The model under review builds one solid part; all positions refer to its coordinate system, in mm. A direction names the side the tool comes from. Give positions to 0.01 mm unless a question says otherwise; leave off trailing zeros. Loops run counter-clockwise (first coordinate to the right, second up) from the corner with the lowest first, then second, coordinate; pieces in that order, holes last. Notation, with made-up numbers: M 21,70 L 46,70 A18 cw 46,87 Z; hole C 14.25,-29.75 d9. An arc over 180 degrees is marked long. Return JSON: item names as keys, results as strings.
```python
from build123d import *

# Parameters (mm, degrees)
SKETCH1_W                       = 112
SKETCH1_H                       = 35.5
BOSS_EXTRUDE1_DEPTH             = 1.2
SKETCH2_W                       = 6
SKETCH2_H                       = 6
BOSS_EXTRUDE2_DEPTH             = 2
SKETCH3_R                       = 1.1
CUT_EXTRUDE1_DEPTH              = 59.83283522
SKETCH5_W                       = 20
SKETCH5_H                       = 14
CUT_EXTRUDE3_DEPTH              = 59.83283522
CHAMFER1_SIZE                   = 0.4
CUT_EXTRUDE6_DEPTH              = 59.779779687
CUT_EXTRUDE6_DEPTH_BACK         = 59.779779687
SKETCH8_W                       = 0.4
SKETCH8_H                       = 35.5
SKIZZE1_W                       = 5.6
SKIZZE1_H                       = 23.5
AUFSATZ_LINEAR_AUSTRAGEN1_DEPTH = 2
SKETCH9_W                       = 5.6
SKETCH9_H                       = 35.5
CUT_EXTRUDE7_DEPTH              = 2
CHAMFER2_SIZE                   = 1.3


with BuildPart() as part:
    # Sketch1 → Boss-Extrude1 (new body)
    with BuildSketch(Plane.XY):
        Rectangle(SKETCH1_W, SKETCH1_H)
    extrude(amount=BOSS_EXTRUDE1_DEPTH)

    # Sketch2 → Boss-Extrude2 (add)
    with BuildSketch(Plane.XY.offset(1.2)):
        with Locations((-53, 14.75)):
            Rectangle(SKETCH2_W, SKETCH2_H)
        with Locations((-53, -14.75)):
            Rectangle(SKETCH2_W, SKETCH2_H)
        with Locations((53, -14.75)):
            Rectangle(SKETCH2_W, SKETCH2_H)
        with Locations((53, 14.75)):
            Rectangle(SKETCH2_W, SKETCH2_H)
    extrude(amount=BOSS_EXTRUDE2_DEPTH)

    # Sketch3 → Cut-Extrude1 (cut, through all)
    with BuildSketch(Plane.XY.offset(3.2)):
        with Locations((-53, 14.75)):
            Circle(SKETCH3_R)
        with Locations((-53, -14.75)):
            Circle(SKETCH3_R)
        with Locations((53, -14.75)):
            Circle(SKETCH3_R)
        with Locations((53, 14.75)):
            Circle(SKETCH3_R)
    extrude(amount=-CUT_EXTRUDE1_DEPTH, mode=Mode.SUBTRACT)

    # Sketch5 → Cut-Extrude3 (cut, through all)
    with BuildSketch(Plane(origin=(0, 0, 0), x_dir=(-1, 0, 0), z_dir=(0, 0, -1))):
        with Locations((29.95, 6.75)):
            Rectangle(SKETCH5_W, SKETCH5_H)
    extrude(amount=-CUT_EXTRUDE3_DEPTH, mode=Mode.SUBTRACT)

    # Chamfer1
    chamfer1_edges = [part.edges().sort_by_distance(p)[0] for p in [
        (-39.95, 6.75, 0),
        (-29.95, 13.75, 0),
        (-19.95, 6.75, 0),
        (-29.95, -0.25, 0),
    ]]
    chamfer(chamfer1_edges, length=CHAMFER1_SIZE)

    # Sketch8 → Cut-Extrude6 (cut, two sides: drawn at the far end of the back side and taken through both)
    with BuildSketch(Plane.XY.offset(1.2).offset(-CUT_EXTRUDE6_DEPTH_BACK)):
        with Locations((-55.8, 0)):
            Rectangle(SKETCH8_W, SKETCH8_H)
        with Locations((55.8, 0)):
            Rectangle(SKETCH8_W, SKETCH8_H)
    extrude(amount=CUT_EXTRUDE6_DEPTH + CUT_EXTRUDE6_DEPTH_BACK, mode=Mode.SUBTRACT)

    # Skizze1 → Aufsatz-Linear austragen1 (add)
    with BuildSketch(Plane.XY.offset(1.2)):
        Polygon((50, -8.156810447), (-50, -8.156810447), (-50, -11.75), (-50, -17.75), (50, -17.75), (50, -11.75), align=None)
        with Locations((-52.8, 0)):
            Rectangle(SKIZZE1_W, SKIZZE1_H)
        with Locations((52.8, 0)):
            Rectangle(SKIZZE1_W, SKIZZE1_H)
    extrude(amount=AUFSATZ_LINEAR_AUSTRAGEN1_DEPTH)

    # Sketch9 → Cut-Extrude7 (cut)
    with BuildSketch(Plane.XY.offset(1.2)):
        with Locations((-52.8, 0)):
            Rectangle(SKETCH9_W, SKETCH9_H)
        with Locations((52.8, 0)):
            Rectangle(SKETCH9_W, SKETCH9_H)
    extrude(amount=CUT_EXTRUDE7_DEPTH, mode=Mode.SUBTRACT)

    # Chamfer2
    # the kernel refuses this chamfer: 1.3 mm, written as the material it takes off along each edge
    with BuildSketch(Plane(origin=(-53, 14.75, 0), x_dir=(1, 0, 0), z_dir=(0, -1, 0))) as chamfer2_piece_1:
        Polygon((1.1 + CHAMFER2_SIZE, 0), (1.1, CHAMFER2_SIZE), (1.1, 0), align=None)
    revolve(axis=Axis((-53, 14.75, 0), (0, 0, 1)), mode=Mode.SUBTRACT)
    with BuildSketch(Plane(origin=(-53, -14.75, 0), x_dir=(1, 0, 0), z_dir=(0, -1, 0))) as chamfer2_piece_2:
        Polygon((1.1 + CHAMFER2_SIZE, 0), (1.1, CHAMFER2_SIZE), (1.1, 0), align=None)
    revolve(axis=Axis((-53, -14.75, 0), (0, 0, 1)), mode=Mode.SUBTRACT)
    with BuildSketch(Plane(origin=(53, -14.75, 0), x_dir=(1, 0, 0), z_dir=(0, -1, 0))) as chamfer2_piece_3:
        Polygon((1.1 + CHAMFER2_SIZE, 0), (1.1, CHAMFER2_SIZE), (1.1, 0), align=None)
    revolve(axis=Axis((53, -14.75, 0), (0, 0, 1)), mode=Mode.SUBTRACT)
    with BuildSketch(Plane(origin=(53, 14.75, 0), x_dir=(1, 0, 0), z_dir=(0, -1, 0))) as chamfer2_piece_4:
        Polygon((1.1 + CHAMFER2_SIZE, 0), (1.1, CHAMFER2_SIZE), (1.1, 0), align=None)
    revolve(axis=Axis((53, 14.75, 0), (0, 0, 1)), mode=Mode.SUBTRACT)


solid = part.part
```
1) Consider section C-C on y = 2.5. Write out the cut boundary in (x, z), then the cut area to 3 significant figures.
From the geometry:
{"outline": "M -55.6,0 L -40.35,0 L -39.95,0.4 L -39.95,1.2 L -55.6,1.2 Z; M -19.95,0.4 L -19.55,0 L 55.6,0 L 55.6,1.2 L -19.95,1.2 Z", "area": "109 mm²"}
2) Insertion check: pin 1 (1.6 mm diameter, centred on y = -15, z = 2.5, fed in from -X); pin 2 (1 mm diameter, centred on y = -15, z = 2, fed in from +X); pin 3 (10 mm diameter, centred on x = 10.5, y = 9, fed in from +Z). Each pin has a flat end and moves straight along its axis. Give the tip position at first contact, or say it passes through.
From the geometry:
{"pin 1": "x = -50", "pin 2": "x = 50", "pin 3": "z = 1.2"}
3) Consider section D-D on x = 53. Write out the cut boundary in (y, z).
From the geometry:
{"outline": "M -17.75,0 L -17.15,0 L -15.95,1.2 L -17.75,1.2 Z; M -13.55,1.2 L -12.35,0 L 12.35,0 L 13.55,1.2 Z; M 15.95,1.2 L 17.15,0 L 17.75,0 L 17.75,1.2 Z"}
4) Tool access review of faces 1 (the face through (50, -13, 2)), 2 (the face through (-50, -13, 2)), 3 (the face through (1, -8.157, 2)): name each direction out of +Z, -Z, +X, -X, +Y, -Y from which nothing blocks a thin tool from reaching the whole face with its end or side.
From the geometry:
{"face 1": "+Z, +X, +Y, -Y", "face 2": "+Z, -X, +Y, -Y", "face 3": "+Z, +X, -X, +Y"}
5) Consider section B-B on y = -14.75. Write out the cut boundary in (x, z).
From the geometry:
{"outline": "M -55.6,0 L -55.4,0 L -54.2,1.2 L -55.6,1.2 Z; M -51.8,1.2 L -50.6,0 L 50.6,0 L 51.8,1.2 L 50,1.2 L 50,3.2 L -50,3.2 L -50,1.2 Z; M 54.2,1.2 L 55.4,0 L 55.6,0 L 55.6,1.2 Z"}
6) Wall thickness on L1, parallel to Y at x = -36, z = 0.65; L2, parallel to Z at x = -43.5, y = 6.5; L3, parallel to Y at x = 22, z = 1.4: over which ranges is each line inside the solid? List them lowest first. Write a range as from..to.
From the geometry:
{"L1": "-17.75..-0.25, 13.75..17.75", "L2": "0..1.2", "L3": "-17.75..-8.16"}
7) Consider section A-A on x = -37. Write out the cut boundary in (y, z).
From the geometry:
{"outline": "M -17.75,0 L -0.65,0 L -0.25,0.4 L -0.25,1.2 L -8.16,1.2 L -8.16,3.2 L -17.75,3.2 Z; M 13.75,0.4 L 14.15,0 L 17.75,0 L 17.75,1.2 L 13.75,1.2 Z"}
